Print and shaded views of the part. All mm, measured from the part's lowest x, y and z. A direction names the side the tool comes from. Give positions to 0.01 mm unless a question says otherwise; leave off trailing zeros. Loops run counter-clockwise (first coordinate to the right, second up) from the corner with the lowest first, then second, coordinate; pieces in that order, holes last.
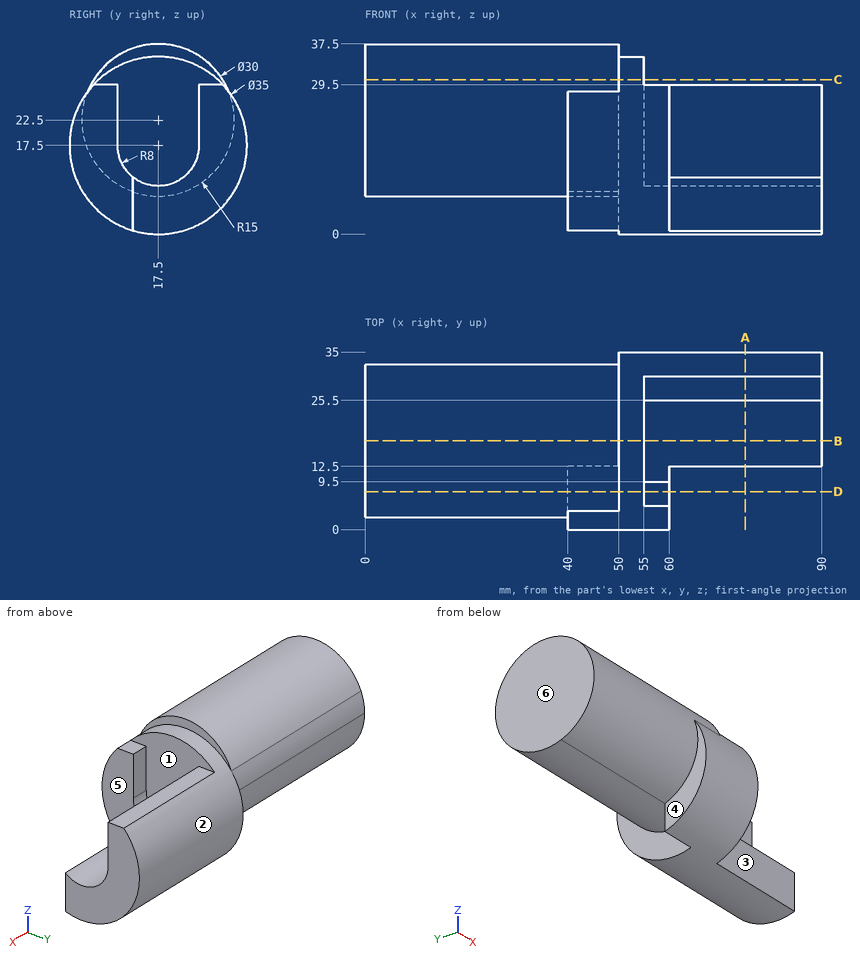
1. Saw through at B-B, the plane y = 17.5. List the corners of the cut face in (x, z).
Responses:
outline: (0, 7.5) - (50, 7.5) - (50, 0) - (90, 0) - (90, 9.5) - (55, 9.5) - (55, 35) - (50, 35) - (50, 37.5) - (0, 37.5) - close
2. Saw through at A-A, the plane x = 75. List the corners of the cut face in (y, z) (1 decimal).
Responses:
outline: (12.5, 0.7) arc R17.5 ccw to (30.2, 29.5) - (25.5, 29.5) - (25.5, 17.5) arc R8 cw to (12.5, 11.3) - close
3. Saw through at D-D, the plane y = 7.5. List the corners of the cut face in (x, z), and give its area (3 significant figures).
Responses:
outline: (0, 11.32) - (40, 11.32) - (40, 3.14) - (60, 3.14) - (60, 29.5) - (55, 29.5) - (55, 31.86) - (50, 31.86) - (50, 33.68) - (0, 33.68) - close
area: 1,480 mm2
4. Drop flat-ended pins along their axis: pin 1 (2 mm diameter, centred on x = 28, y = 9.5, fed in from -Z); pin 2 (12 mm diameter, centred on x = 64.5, z = 12, fed in from -Y); pin 3 (1.5 mm diameter, centred on x = 57, z = 22, fed in from +Y). Give the stop position or say it passes through.
Responses:
pin 1: stops at z = 9.23
pin 2: stops at y = 0.07
pin 3: stops at y = 34.59
5. Tool access for the marked faces 5 and 6: list every direction of +Z, -Z, +X, -X, +Y, -Y with a clear straight run to the whole face (end or side of a thin tool).
Responses:
face 5: +Z, -Z, +X, -Y
face 6: +Z, -Z, -X, +Y, -Y
6. Probe line 1 along X through (y, z) = (15.5, 4.5); line 2 along X through (y, z) = (7.5, 14.5); line 3 along Z through (x, y) = (79, 26). List the from-to ranges inside material, lowest first.
Responses:
line 1: x = 50 to 90
line 2: x = 0 to 60
line 3: z = 2.2 to 29.5
7. Pull direction Y, two halves, no side cores. Call the marked faces 1, 2, 3 and 4: released by +Y, released by -Y, zero draft, split by the parting line, or undercut.
Responses:
face 1: undercut
face 2: split by the parting line
face 3: released by -Y
face 4: zero draft
8. Saw through at C-C, the plane z = 30.5. List the corners of the cut face in (x, y), and give its area (3 significant figures).
Responses:
outline: (0, 4.81) - (50, 4.81) - (50, 5.78) - (55, 5.78) - (55, 29.22) - (50, 29.22) - (50, 30.19) - (0, 30.19) - close
area: 1,390 mm2
